```python
from build123d import *

# Parameters (mm, degrees)
SKETCH1_R           = 3.96875
EXTRUDE1_DEPTH      = 107.95
CHAMFER1_SIZE       = 0.5953125
EXTRUDE2_DEPTH      = 109.09581145
EXTRUDE2_DEPTH_BACK = 109.09581145
SKETCH3_W           = 2.38125
SKETCH3_H           = 1.190625


with BuildPart() as part:
    # Sketch1 → Extrude1 (new, symmetric)
    with BuildSketch(Plane.XY):
        Circle(SKETCH1_R)
    extrude(amount=EXTRUDE1_DEPTH, both=True)

    # Chamfer1
    chamfer1_edges = [part.edges().sort_by_distance(p)[0] for p in [
        (-3.96875, 0, -107.95),
        (-3.96875, 0, 107.95),
    ]]
    chamfer(chamfer1_edges, length=CHAMFER1_SIZE)

    # Sketch3 → Extrude2 (cut, two sides: drawn at the far end of the back side and taken through both)
    with BuildSketch(Plane.XY.offset(-EXTRUDE2_DEPTH_BACK)):
        with Locations((0, 3.3734375)):
            Rectangle(SKETCH3_W, SKETCH3_H)
    extrude(amount=EXTRUDE2_DEPTH + EXTRUDE2_DEPTH_BACK, mode=Mode.SUBTRACT)


solid = part.part
```
Geometry: final body of the model. Coordinates: model frame, mm. Round coordinates to 2 decimals unless told otherwise and drop trailing zeros. Order: outer loops, then holes, each group sorted by start corner. A loop starts at its lowest first (then second) coordinate and runs counter-clockwise, first axis right, second up. Notation, with made-up numbers: (86.5, 63.25) -> (97.5, 63.25) arc R24 cw to (97.5, 99.25) -> close; hole circle Ø2 at (81.25, -10). An arc over 180 degrees is marked (long way). Use CSV: the item, a comma, the result in double quotes. Start each with the question number.
1) Material intervals for line 1 along X through (y, z) = (3.25, -61.5); line 2 along Y through (x, z) = (-0.5, 88); line 3 along X through (y, z) = (0.5, 67), sorted ascending. Write a range as from..to.
2) Section A-A (z = -33.5). Return the cut outline in (x, y), and give its area (3 significant figures).
3) First-contact query: pin 1 Ø1 at (x, z) = (1, -68) entering from -Y; pin 2 Ø3 at (y, z) = (-3, 64.5) entering from -X; pin 3 Ø1.2 at (x, z) = (0, 20.5) entering from +Y. Flat tips, straight axial feed; report the tip coordinate or a pass-through.
Returned:
1,line 1,"x = -2.28..-1.19, 1.19..2.28"
1,line 2,"y = -3.94..2.78"
1,line 3,"x = -3.94..3.94"
2,outline,"(-1.19, 2.78) -> (-1.19, 3.79) arc R3.97 ccw (long way) to (1.19, 3.79) -> (1.19, 2.78) -> close"
2,area,"46.8 mm²"
3,pin 1,"stops at y = -3.94"
3,pin 2,"stops at x = -3.67"
3,pin 3,"stops at y = 2.78"
